Build history of the part. All positions in model axes, mm. Face numbers are marked on the shaded views. Give positions to 0.01 mm unless a question says otherwise; leave off trailing zeros. Write each loop counter-clockwise with the first axis right and the second up, starting at its lowest first coordinate (ties: lowest second). Pieces come first, ordered by that corner, then holes. Notation, with made-up numbers: (18.5, 1) -> (30.5, 1) arc R16 cw to (30.5, 8) -> close; hole circle Ø10 at (30, 38). An arc over 180 degrees is marked (long way). Put each result on its own line as item: value.
from build123d import *

# Parameters (mm, degrees)
SKETCH1_W           = 20
SKETCH1_H           = 25
BOSS_EXTRUDE1_DEPTH = 5
CUT_EXTRUDE1_REACH  = 7
SKETCH3_R           = 6.35
SKETCH5_R           = 0.75
CUT_EXTRUDE2_DEPTH  = 7
CUT_EXTRUDE3_REACH  = 22
SKETCH6_R           = 1.25


with BuildPart() as part:
    # Sketch1 → Boss-Extrude1 (new body)
    with BuildSketch(Plane.XY):
        with Locations((-14.085851727, 19.333014081)):
            Rectangle(SKETCH1_W, SKETCH1_H)
    extrude(amount=BOSS_EXTRUDE1_DEPTH)

    # Sketch3 → Cut-Extrude1 (cut, up to next)
    with BuildSketch(Plane.XY.offset(5), mode=Mode.PRIVATE) as cut_extrude1_sk1:
        with Locations((-14.085851727, 14.333014081)):
            Circle(SKETCH3_R)
    cut_extrude1_tool1 = extrude(cut_extrude1_sk1.sketch, amount=-CUT_EXTRUDE1_REACH, mode=Mode.PRIVATE) & part.part
    add(cut_extrude1_tool1.solids().sort_by_distance((-14.085852, 14.333014, 5))[0], mode=Mode.SUBTRACT)

    # Sketch5 → Cut-Extrude2 (cut)
    with BuildSketch(Plane(origin=(0, 31.833014081, 0), x_dir=(1, 0, 0), z_dir=(0, 1, 0))):
        with Locations((-10.085851727, -2.5)):
            Circle(SKETCH5_R)
        with Locations((-18.085851727, -2.5)):
            Circle(SKETCH5_R)
    extrude(amount=-CUT_EXTRUDE2_DEPTH, mode=Mode.SUBTRACT)

    # Sketch6 → Cut-Extrude3 (cut, up to next)
    with BuildSketch(Plane(origin=(-4.085851727, 0, 0), x_dir=(0, 0, -1), z_dir=(1, 0, 0)), mode=Mode.PRIVATE) as cut_extrude3_sk1:
        with Locations((-2.5, 14.333014081)):
            Circle(SKETCH6_R)
    cut_extrude3_tool1 = extrude(cut_extrude3_sk1.sketch, amount=-CUT_EXTRUDE3_REACH, mode=Mode.PRIVATE) & part.part
    add(cut_extrude3_tool1.solids().sort_by_distance((-4.085852, 14.333014, 2.5))[0], mode=Mode.SUBTRACT)


solid = part.part
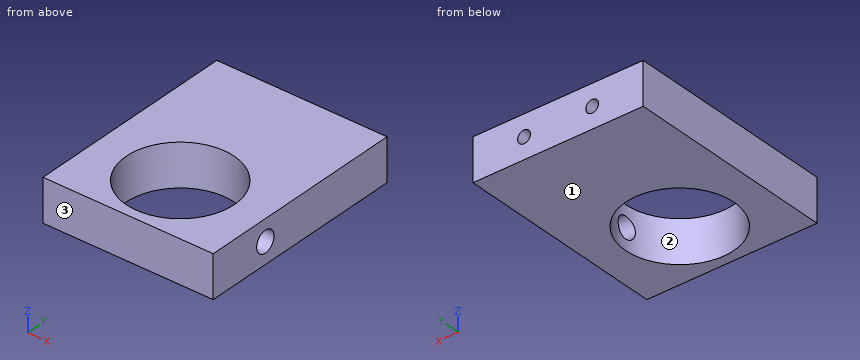
1) Wall check: L1, parallel to X at y = 27, z = 2.5; L2, parallel to Z at x = -18, y = 27.75; L3, parallel to Y at x = -5.5, z = 2.5. Give the ranges that are in metal, low to high.
Filled sheet:
L1: -24.09 to -18.84, -17.34 to -10.84, -9.34 to -4.09
L2: 0 to 1.75, 3.25 to 5
L3: 6.83 to 13.08, 15.58 to 31.83
2) Slice it at D-D (x = -5.75). Write the cut outline in (y, z).
Filled sheet:
outline: (6.83, 0) -> (31.83, 0) -> (31.83, 5) -> (6.83, 5) -> close; hole circle Ø2.5 at (14.33, 2.5)
3) Slice it at A-A (x = -19.5). Write the cut outline in (y, z), plus the area to 3 significant figures.
Filled sheet:
outline: (6.83, 0) -> (11.01, 0) -> (11.01, 5) -> (6.83, 5) -> close; (17.65, 0) -> (31.83, 0) -> (31.83, 5) -> (17.65, 5) -> close
area: 91.8 mm2
4) Slice it at B-B (z = 2.5). Write the cut outline in (x, y), plus the area to 3 significant figures.
Filled sheet:
outline: (-24.09, 6.83) -> (-4.09, 6.83) -> (-4.09, 13.08) -> (-7.86, 13.08) arc R6.35 cw (long way) to (-7.86, 15.58) -> (-4.09, 15.58) -> (-4.09, 31.83) -> (-9.34, 31.83) -> (-9.34, 24.83) -> (-10.84, 24.83) -> (-10.84, 31.83) -> (-17.34, 31.83) -> (-17.34, 24.83) -> (-18.84, 24.83) -> (-18.84, 31.83) -> (-24.09, 31.83) -> close
area: 343 mm2
5) Pull direction Y, two halves, no side cores. Call the marked faces 1, 2 and 3: released by +Y, released by -Y, zero draft, split by the parting line, or undercut.
Filled sheet:
face 1: zero draft
face 2: undercut
face 3: released by -Y
6) Slice it at C-C (y = 9). Write the cut outline in (x, z), plus the area to 3 significant figures.
Filled sheet:
outline: (-24.09, 0) -> (-17.53, 0) -> (-17.53, 5) -> (-24.09, 5) -> close; (-10.64, 0) -> (-4.09, 0) -> (-4.09, 5) -> (-10.64, 5) -> close
area: 65.5 mm2
